Part model, mm, in its own coordinate system. Coordinates: 2 decimals unless noted, no trailing zeros. Order: outer loops, then holes, each group sorted by start corner. A loop starts at its lowest first (then second) coordinate and runs counter-clockwise, first axis right, second up. Notation, with made-up numbers: (40.25, -38) - (72.25, -38) arc R12 ccw to (72.25, -31) - close; hole circle Ø6 at (46, 63). An arc over 180 degrees is marked (long way). Use a Markdown table: item, result. Add a question column.
1) Saw through at A-A on z = 6. List the corners of the cut face in (x, y), then the cut area to 3 significant figures.
2) Drop a flat-ended pin along its axis: P1, Ø5, axis at x = 3, z = -2.5, coming from the -Y side. Give the stop position or say it passes through.
3) Wall check: L1, parallel to Z at x = 5.5, y = 0.4; L2, parallel to X at y = 0.1, z = -1.5; L3, parallel to Z at x = 4, y = 0.15. Give the ranges that are in metal, low to high. Write a range as [from, to].
4) Saw through at B-B on x = -2.25. List the corners of the cut face in (y, z), then the cut area to 3 significant figures.
5) Saw through at D-D on z = -4.5. List the corners of the cut face in (x, y).
6) Saw through at C-C on y = 0.3. Count the separate pieces of the cut face and the enclosed holes in it, then the cut area to 3 significant figures.
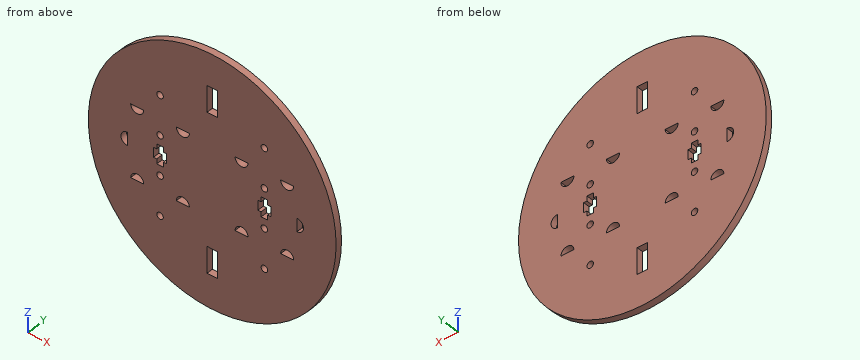
```python
from build123d import *

# Parameters (mm, degrees)
SKETCH1_R      = 9.5
SKETCH1_R_2    = 0.25
SKETCH1_W      = 0.8
SKETCH1_H      = 2
EXTRUDE1_DEPTH = 0.5
SKETCH2_R      = 0.25
EXTRUDE2_DEPTH = 1.5


with BuildPart() as part:
    # Sketch1 → Extrude1 (new body)
    with BuildSketch(Plane(origin=(0, 0, 0), x_dir=(1, 0, 0), z_dir=(0, 1, 0))):
        Circle(SKETCH1_R)
        with Locations((-4, 4.5)):
            Circle(SKETCH1_R_2, mode=Mode.SUBTRACT)
        with Locations((4, 4.5)):
            Circle(SKETCH1_R_2, mode=Mode.SUBTRACT)
        with Locations((4, -4.5)):
            Circle(SKETCH1_R_2, mode=Mode.SUBTRACT)
        with Locations((-4, -4.5)):
            Circle(SKETCH1_R_2, mode=Mode.SUBTRACT)
        with Locations((0, 6)):
            Rectangle(SKETCH1_W, SKETCH1_H, mode=Mode.SUBTRACT)
        with Locations((0, -6)):
            Rectangle(SKETCH1_W, SKETCH1_H, mode=Mode.SUBTRACT)
    extrude(amount=EXTRUDE1_DEPTH)

    # Sketch2 → Extrude2 (cut, through all)
    with BuildSketch(Plane(origin=(0, 0, 0), x_dir=(1, 0, 0), z_dir=(0, 1, 0))):
        with Locations((4, 1.5)):
            Circle(SKETCH2_R)
        with Locations((4, -1.5)):
            Circle(SKETCH2_R)
        with Locations((-4, 1.5)):
            Circle(SKETCH2_R)
        with Locations((-4, -1.5)):
            Circle(SKETCH2_R)
        Polygon((3.75, 0.75), (4.25, 0.75), (4.25, 0.375), (4.5, 0.375), (4.5, -0.375), (4.25, -0.375), (4.25, -0.75), (3.75, -0.75), (3.75, -0.375), (3.5, -0.375), (3.5, 0.375), (3.75, 0.375), align=None)
        Polygon((-3.5, 0.375), (-3.5, -0.375), (-3.75, -0.375), (-3.75, -0.75), (-4.25, -0.75), (-4.25, -0.375), (-4.5, -0.375), (-4.5, 0.375), (-4.25, 0.375), (-4.25, 0.75), (-3.75, 0.75), (-3.75, 0.375), align=None)
        with BuildLine():
            Line((-6.5, 0.5), (-6.5, -0.5))
            ThreePointArc((-6.5, -0.5), (-7, 0), (-6.5, 0.5))
        make_face()
        with BuildLine():
            Line((6.5, 0.5), (6.5, -0.5))
            ThreePointArc((6.5, -0.5), (7, 0), (6.5, 0.5))
        make_face()
        with BuildLine():
            Line((-6.25, 2.75), (-5.25, 2.75))
            ThreePointArc((-5.25, 2.75), (-5.75, 2.25), (-6.25, 2.75))
        make_face()
        with BuildLine():
            Line((-2.75, 2.75), (-1.75, 2.75))
            ThreePointArc((-1.75, 2.75), (-2.25, 2.25), (-2.75, 2.75))
        make_face()
        with BuildLine():
            Line((1.75, 2.75), (2.75, 2.75))
            ThreePointArc((2.75, 2.75), (2.25, 2.25), (1.75, 2.75))
        make_face()
        with BuildLine():
            Line((5.25, 2.75), (6.25, 2.75))
            ThreePointArc((6.25, 2.75), (5.75, 2.25), (5.25, 2.75))
        make_face()
        with BuildLine():
            Line((-6.25, -2.75), (-5.25, -2.75))
            ThreePointArc((-5.25, -2.75), (-5.75, -2.25), (-6.25, -2.75))
        make_face()
        with BuildLine():
            Line((-2.75, -2.75), (-1.75, -2.75))
            ThreePointArc((-1.75, -2.75), (-2.25, -2.25), (-2.75, -2.75))
        make_face()
        with BuildLine():
            Line((1.75, -2.75), (2.75, -2.75))
            ThreePointArc((2.75, -2.75), (2.25, -2.25), (1.75, -2.75))
        make_face()
        with BuildLine():
            Line((5.25, -2.75), (6.25, -2.75))
            ThreePointArc((6.25, -2.75), (5.75, -2.25), (5.25, -2.75))
        make_face()
    extrude(amount=EXTRUDE2_DEPTH, mode=Mode.SUBTRACT)


solid = part.part
```
Results are:
| question | item | result |
|---|---|---|
| 1 | outline | (-7.37, 0) - (-0.4, 0) - (-0.4, 0.5) - (-7.37, 0.5) - close; (0.4, 0) - (7.37, 0) - (7.37, 0.5) - (0.4, 0.5) - close |
| 1 | area | 6.97 mm2 |
| 2 | P1 | y = 0 |
| 3 | L1 | [-7.75, -2.75], [-2.32, 2.32], [2.75, 7.75] |
| 3 | L2 | [-9.38, -4.25], [-3.75, 3.75], [4.25, 9.38] |
| 3 | L3 | [-8.62, -4.75], [-4.25, -1.75], [-1.25, -0.75], [0.75, 1.25], [1.75, 4.25], [4.75, 8.62] |
| 4 | outline | (0, -9.23) - (0.5, -9.23) - (0.5, -2.75) - (0, -2.75) - close; (0, -2.25) - (0.5, -2.25) - (0.5, 2.25) - (0, 2.25) - close; (0, 2.75) - (0.5, 2.75) - (0.5, 9.23) - (0, 9.23) - close |
| 4 | area | 8.73 mm2 |
| 5 | outline | (-8.37, 0) - (-4.25, 0) - (-4.25, 0.5) - (-8.37, 0.5) - close; (-3.75, 0) - (3.75, 0) - (3.75, 0.5) - (-3.75, 0.5) - close; (4.25, 0) - (8.37, 0) - (8.37, 0.5) - (4.25, 0.5) - close |
| 6 | separate pieces | 1 |
| 6 | enclosed holes | 22 |
| 6 | area | 273 mm2 |
